```python
from build123d import *

# Parameters (mm, degrees)
RESSALTO_EXTRUS_O1_DEPTH   = 160
ESBO_O2_W                  = 7.6
ESBO_O2_H                  = 120
CORTE_EXTRUS_O1_DEPTH      = 30
CORTE_EXTRUS_O2_DEPTH      = 30
F_3DSKETCH3_R              = 2
CORTE_EXTRUS_O3_DEPTH      = 70
ESBO_O3_W                  = 45.015344868
ESBO_O3_H                  = 129.478543367
ESBO_O3_W_2                = 37.192593828
CORTE_EXTRUS_O4_DEPTH      = 41
CORTE_EXTRUS_O4_DEPTH_BACK = 22


with BuildPart() as part:
    # Esboço1 → Ressalto-extrusão1 (new body)
    with BuildSketch(Plane.XY):
        with BuildLine():
            Line((-3.8, 21.821375341), (-3.8, -98.178624659))
            Line((-3.8, -98.178624659), (-5.7, -98.178624659))
            Line((-5.7, -98.178624659), (-5.360626179, -99.63308389))
            ThreePointArc((-5.360626179, -99.63308389), (-4.656141559, -100.745296045), (-3.41294376, -101.178624659))
            Line((-3.41294376, -101.178624659), (3.41294376, -101.178624659))
            ThreePointArc((3.41294376, -101.178624659), (4.656141559, -100.745296045), (5.360626179, -99.63308389))
            Line((5.360626179, -99.63308389), (5.7, -98.178624659))
            Line((5.7, -98.178624659), (3.8, -98.178624659))
            Line((3.8, -98.178624659), (3.8, 21.821375341))
            Line((3.8, 21.821375341), (5.7, 21.821375341))
            Line((5.7, 21.821375341), (4.013268169, 24.033911877))
            ThreePointArc((4.013268169, 24.033911877), (3.310139149, 24.613730366), (2.422747768, 24.821375341))
            Line((2.422747768, 24.821375341), (-2.297792791, 24.821375341))
            ThreePointArc((-2.297792791, 24.821375341), (-3.27177376, 24.568189891), (-3.999156919, 23.872736414))
            Line((-3.999156919, 23.872736414), (-5.266799243, 21.821375341))
            Line((-5.266799243, 21.821375341), (-3.8, 21.821375341))
        make_face()
    extrude(amount=RESSALTO_EXTRUS_O1_DEPTH)

    # Esboço2 → Corte-extrusão1 (cut)
    with BuildSketch(Plane.XY):
        with Locations((0, -38.178624659)):
            Rectangle(ESBO_O2_W, ESBO_O2_H)
    extrude(amount=CORTE_EXTRUS_O1_DEPTH, mode=Mode.SUBTRACT)

    # 3DSketch2 → Corte-extrusão2 (cut)
    with BuildSketch(Plane(origin=(-3.8, 21.821375341, 160), x_dir=(0.0632066956560733, -0.9980004577274705, 0), z_dir=(0, 0, -1))):
        Polygon((0, 0), (0.480370887, -7.584803479), (120.240425814, 0), (119.760054927, 7.584803479), align=None)
    extrude(amount=CORTE_EXTRUS_O2_DEPTH, mode=Mode.SUBTRACT)

    # 3DSketch3 → Corte-extrusão3 (cut)
    with BuildSketch(Plane(origin=(3.8, -38.178624659, 80), x_dir=(0, 0.7676852805184269, 0.6408270516101394), z_dir=(1, 0, 0))):
        with Locations(Location((0, 0, 0), (0, 0, 140.146481665))):
            Circle(F_3DSKETCH3_R)
        with Locations(Location((23.030558416, -19.224811548, 0), (0, 0, 140.146481665))):
            Circle(F_3DSKETCH3_R)
        with Locations(Location((-23.030558416, 19.224811548, 0), (0, 0, 140.146481665))):
            Circle(F_3DSKETCH3_R)
        with Locations(Location((-39.051234706, 0.032679535, 0), (0, 0, 140.146481665))):
            Circle(F_3DSKETCH3_R)
        with Locations(Location((-16.02067629, -19.192132013, 0), (0, 0, 140.146481665))):
            Circle(F_3DSKETCH3_R)
        with Locations(Location((7.009882125, -38.416943561, 0), (0, 0, 140.146481665))):
            Circle(F_3DSKETCH3_R)
        with Locations(Location((-6.982602808, 38.449623097, 0), (0, 0, 140.146481665))):
            Circle(F_3DSKETCH3_R)
        with Locations(Location((16.047955607, 19.224811548, 0), (0, 0, 140.146481665))):
            Circle(F_3DSKETCH3_R)
        with Locations(Location((39.078514023, 0, 0), (0, 0, 140.146481665))):
            Circle(F_3DSKETCH3_R)
    extrude(amount=-CORTE_EXTRUS_O3_DEPTH, mode=Mode.SUBTRACT)

    # Esboço3 → Corte-extrusão4 (cut, two sides)
    with BuildSketch(Plane(origin=(0, 0, 0), x_dir=(0, 0, -1), z_dir=(1, 0, 0))) as corte_extrus_o4_sk:
        with Locations((-7.492327566, -39.917896343)):
            Rectangle(ESBO_O3_W, ESBO_O3_H)
        with Locations((-148.596296914, -39.917896343)):
            Rectangle(ESBO_O3_W_2, ESBO_O3_H)
    extrude(amount=CORTE_EXTRUS_O4_DEPTH, mode=Mode.SUBTRACT)
    extrude(corte_extrus_o4_sk.sketch, amount=-CORTE_EXTRUS_O4_DEPTH_BACK, mode=Mode.SUBTRACT)


solid = part.part
```
Geometry check sheet. Reference: the model listing, model coordinates, mm. A direction names the side the tool comes from. Round coordinates to 2 decimals unless told otherwise and drop trailing zeros. Write each loop counter-clockwise with the first axis right and the second up, starting at its lowest first coordinate (ties: lowest second). Pieces come first, ordered by that corner, then holes. Notation, with made-up numbers: (16, 38.5) -> (31, 38.5) arc R20 cw to (31, 51.5) -> close; hole circle Ø5 at (-12.75, 41.5). An arc over 180 degrees is marked (long way). Put each result on its own line as item: value.
1) Thickness scan on probe 1 along Z at (x, y) = (1, -38); probe 2 along X at (y, z) = (-19, 57); probe 3 along Y at (x, z) = (-2.5, 107.5). Record the ranges inside material, lowest first. Write a range as from..to.
Recorded:
probe 1: z = 30..53.01, 56.99..78.01, 81.99..103.05, 107.03..130
probe 2: x = -3.8..3.8
probe 3: y = -101.18..24.81
2) Cross-section at B-B, the plane z = 101. Enter the section's corners in (x, y), plus the area to 3 significant figures.
Recorded:
outline: (-5.7, -98.18) -> (-5.36, -99.63) arc R2 ccw to (-3.41, -101.18) -> (3.41, -101.18) arc R2 ccw to (5.36, -99.63) -> (5.7, -98.18) -> (3.8, -98.18) -> (3.8, 21.82) -> (5.7, 21.82) -> (4.01, 24.03) arc R2 ccw to (2.42, 24.82) -> (-2.3, 24.82) arc R2 ccw to (-4, 23.87) -> (-5.27, 21.82) -> (-3.8, 21.82) -> (-3.8, -98.18) -> close
area: 969 mm2
3) Depth check by flat-ended pin: P1, Ø3, axis at y = -8.18, z = 80, coming from the -X side; P2, Ø8, axis at y = 0.5, z = 107.5, coming from the -X side; P3, Ø1.2, axis at x = -4.5, z = 73, coming from the -Y side; P4, Ø0.6, axis at x = -5, z = 85, coming from the +Y side. Enter the tip coordinate at first touch or a pass-through.
Recorded:
P1: passes through
P2: stops at x = -3.8
P3: stops at y = -101.12
P4: stops at y = 22.74
4) Cross-section at C-C, the plane y = 15. Enter the section's corners in (x, z).
Recorded:
outline: (-3.8, 30) -> (3.8, 30) -> (3.8, 130) -> (-3.8, 130) -> close
5) Access from +Z, -Z, +X, -X, +Y, -Y to the whole of each face (thin tool, end or side, straight path). Record for faces 4 (the face through (3.8, -39, 68)), 5 (the face through (0.05, -37.92, 103.06)), 6 (the face through (-3.8, -37, 68)).
Recorded:
face 4: +Z, -Z, +X
face 5: +X, -X
face 6: +Z, -Z, -X
6) Cross-section at A-A, the plane z = 80. Enter the section's corners in (x, y).
Recorded:
outline: (-5.7, -98.18) -> (-5.36, -99.63) arc R2 ccw to (-3.41, -101.18) -> (3.41, -101.18) arc R2 ccw to (5.36, -99.63) -> (5.7, -98.18) -> (3.8, -98.18) -> (3.8, -70.18) -> (-3.8, -70.18) -> (-3.8, -98.18) -> close; (-5.27, 21.82) -> (-3.8, 21.82) -> (-3.8, -6.18) -> (3.8, -6.18) -> (3.8, 21.82) -> (5.7, 21.82) -> (4.01, 24.03) arc R2 ccw to (2.42, 24.82) -> (-2.3, 24.82) arc R2 ccw to (-4, 23.87) -> close; (-3.8, -66.18) -> (3.8, -66.18) -> (3.8, -40.18) -> (-3.8, -40.18) -> close; (-3.8, -36.18) -> (3.8, -36.18) -> (3.8, -10.18) -> (-3.8, -10.18) -> close
7) Release check for a two-part mould opening along Z. For faces 1 (the face through (0, 24.821, 79)), 2 (the face through (0.053, -7.745, 56.952)), 3 (the face through (-1, -39, 130)) record: pulls with the +Z half, pulls with the -Z half, needs draft (parallel to the pull), parting line crosses it, or undercut.
Recorded:
face 1: needs draft
face 2: undercut
face 3: pulls with the +Z half
